Part model, mm, in its own coordinate system. A direction names the side the tool comes from. Coordinates: 2 decimals unless noted, no trailing zeros.
```python
from build123d import *

# Parameters (mm, degrees)
BOSS_EXTRUDE1_DEPTH            = 55.88
BOSS_EXTRUDE1_DEPTH_BACK       = 144.78
SKETCH1_W                      = 12.7
SKETCH1_H                      = 12.7
F_5_16_0_3125_DIAMETER_HOLE2_D = 7.9375
SKETCH9_W                      = 6.604
SKETCH9_H                      = 12.7
CUT_EXTRUDE1_DEPTH             = 19.05
SKETCH19_W                     = 3.2004
SKETCH19_H                     = 12.7
CUT_EXTRUDE2_DEPTH             = 12.7
ADVANCEDHOLE2_START            = 5.08
ADVANCEDHOLE2_OUTLINE_R        = 3.302
ADVANCEDHOLE2_DEPTH            = 1.27
ADVANCEDHOLE2_START_2          = -6.35
ADVANCEDHOLE2_2_OUTLINE_R      = 1.1303
ADVANCEDHOLE2_2_DEPTH          = 11.43
ADVANCEDHOLE2_START_3          = 1.6002
ADVANCEDHOLE2_3_OUTLINE_R      = 1.6002
ADVANCEDHOLE2_3_OUTLINE_R_2    = 1.1303
ADVANCEDHOLE2_3_DEPTH          = 3.4798
CUT_EXTRUDE3_DEPTH             = 3.175


# Read off the part's stored shape, not the designer's step: AdvancedHole2
with BuildPart() as part:
    # Sketch1 → Boss-Extrude1 (new, two sides: drawn at the far end of the back side and taken through both)
    with BuildSketch(Plane(origin=(0, 0, 0), x_dir=(0, 0, -1), z_dir=(1, 0, 0)).offset(-BOSS_EXTRUDE1_DEPTH_BACK)):
        Rectangle(SKETCH1_W, SKETCH1_H)
    extrude(amount=BOSS_EXTRUDE1_DEPTH + BOSS_EXTRUDE1_DEPTH_BACK)

    # 5/16 (0.3125) Diameter Hole2 (through all)
    with Locations(Plane.XY.offset(6.35)):
        with Locations((0, 0)):
            Hole(F_5_16_0_3125_DIAMETER_HOLE2_D / 2)

    # Sketch9 → Cut-Extrude1 (cut)
    with BuildSketch(Plane(origin=(55.88, 0, 0), x_dir=(0, 0, -1), z_dir=(1, 0, 0))):
        Rectangle(SKETCH9_W, SKETCH9_H)
    extrude(amount=-CUT_EXTRUDE1_DEPTH, mode=Mode.SUBTRACT)

    # Sketch19 → Cut-Extrude2 (cut)
    with BuildSketch(Plane.ZY.offset(144.78)):
        Rectangle(SKETCH19_W, SKETCH19_H)
    extrude(amount=-CUT_EXTRUDE2_DEPTH, mode=Mode.SUBTRACT)

    # AdvancedHole2 outline → AdvancedHole2 (cut)
    with BuildSketch(Plane.XY.offset(ADVANCEDHOLE2_START)):
        with Locations((-138.43, 0)):
            Circle(ADVANCEDHOLE2_OUTLINE_R)
        with Locations((49.53, 0)):
            Circle(ADVANCEDHOLE2_OUTLINE_R)
    extrude(amount=ADVANCEDHOLE2_DEPTH, mode=Mode.SUBTRACT)

    # AdvancedHole2 2 outline → AdvancedHole2 2 (cut)
    with BuildSketch(Plane.XY.offset(ADVANCEDHOLE2_START_2)):
        with Locations((-138.43, 0)):
            Circle(ADVANCEDHOLE2_2_OUTLINE_R)
        with Locations((49.53, 0)):
            Circle(ADVANCEDHOLE2_2_OUTLINE_R)
    extrude(amount=ADVANCEDHOLE2_2_DEPTH, mode=Mode.SUBTRACT)

    # AdvancedHole2 3 outline → AdvancedHole2 3 (cut)
    # profile 1 of 2: a face of its own
    with BuildSketch(Plane.XY.offset(ADVANCEDHOLE2_START_3)):
        with Locations((-138.43, 0)):
            Circle(ADVANCEDHOLE2_3_OUTLINE_R)
        with Locations((-138.43, 0)):
            Circle(ADVANCEDHOLE2_3_OUTLINE_R_2, mode=Mode.SUBTRACT)
    # profile 2 of 2: a face of its own
    with BuildSketch(Plane.XY.offset(ADVANCEDHOLE2_START_3)):
        with Locations((49.53, 0)):
            Circle(ADVANCEDHOLE2_3_OUTLINE_R)
        with Locations((49.53, 0)):
            Circle(ADVANCEDHOLE2_3_OUTLINE_R_2, mode=Mode.SUBTRACT)
    extrude(amount=ADVANCEDHOLE2_3_DEPTH, mode=Mode.SUBTRACT)

    # Sketch20 → Cut-Extrude3 (cut)
    with BuildSketch(Plane(origin=(0, 6.35, 0), x_dir=(1, 0, 0), z_dir=(0, 1, 0))):
        with BuildLine():
            Line((36.83, -3.302), (8.89, -3.302))
            ThreePointArc((8.89, -3.302), (5.588, 0), (8.89, 3.302))
            Line((8.89, 3.302), (36.83, 3.302))
            ThreePointArc((36.83, 3.302), (40.132, 0), (36.83, -3.302))
        make_face()
    extrude(amount=-CUT_EXTRUDE3_DEPTH, mode=Mode.SUBTRACT)


solid = part.part
```
(1) Drop flat-ended pins along their axis: pin 1 (2 mm diameter, centred on x = -137, y = -1, fed in from +Z); pin 2 (2 mm diameter, centred on y = 2.5, z = 0, fed in from -X); pin 3 (3.5 mm diameter, centred on x = 26, z = -0.5, fed in from +Y) (3 decimals). Give the stop position or say it passes through.
(2) Tool access for faces 4 (the face through (-132.08, 0, 0)), 5 (the face through (43, 1, -3.302)), 6 (the face through (47.93, 0.07, 4.18)), 7 (the face through (36.83, -2, 0)): list every direction of +Z, -Z, +X, -X, +Y, -Y with a clear straight run to the whole face (end or side of a thin tool).
(3) Pull direction Z, two halves, no side cores. Call faces 1 (the face through (-46, -6.35, 0)), 2 (the face through (-46, 0, 6.35)), 3 (the face through (-140, 0, -1.6)): +Z half, -Z half, draft (parallel to the pull), parting line (faces both ways), or undercut.
(4) Probe line 1 (X direction, y = -0.25, z = -4.5); line 2 (Y direction, x = -138.43, z = 6). List the from-to ranges inside material, lowest first.
Here are the results:
1. pin 1: stops at z = 5.08
1. pin 2: stops at x = -132.08
1. pin 3: stops at y = 3.175
2. face 4: -X, +Y, -Y
2. face 5: +X, +Y
2. face 6: +Z
2. face 7: +X, +Y, -Y
3. face 1: draft
3. face 2: +Z half
3. face 3: undercut
4. line 1: x = -144.78 to -139.53, -137.33 to -3.96, 3.96 to 48.43, 50.63 to 55.88
4. line 2: y = -6.35 to -3.3, 3.3 to 6.35
